The listing builds one solid part. Answer for the finished solid, in the listing's coordinates (mm). A direction names the side the tool comes from. Coordinates: 2 decimals unless noted, no trailing zeros. Write each loop counter-clockwise with the first axis right and the second up, starting at its lowest first coordinate (ties: lowest second). Pieces come first, ordered by that corner, then holes. Notation, with made-up numbers: M 63,82 L 83,82 A31 cw 83,120 Z; hole C 61,-10.5 d10. An arc over 180 degrees is marked long. Answer as CSV lines item,"result". Start each with the question number.
```python
from build123d import *

# Parameters (mm, degrees)
SKETCH1_R           = 9.525
BOSS_EXTRUDE1_DEPTH = 7.62


with BuildPart() as part:
    # Sketch1 → Boss-Extrude1 (new body)
    with BuildSketch(Plane(origin=(0, 0, 0), x_dir=(1, 0, 0), z_dir=(0, 1, 0))):
        with BuildLine():
            Line((-4.826, 49.377023111), (-4.826, 76.047023111))
            ThreePointArc((-4.826, 76.047023111), (-8.902418576, 75.678180102), (-12.953151139, 75.090983983))
            ThreePointArc((-12.953151139, 75.090983983), (-31.496, 54.552672235), (-58.554124155, 48.763249937))
            ThreePointArc((-58.554124155, 48.763249937), (-61.088017192, 45.548810693), (-63.445653896, 42.202950154))
            Line((-63.445653896, 42.202950154), (-40.348756377, 28.867950154))
            ThreePointArc((-40.348756377, 28.867950154), (-38.582317778, 22.275511555), (-45.174756377, 20.509072957))
            Line((-45.174756377, 20.509072957), (-68.271653896, 33.844072957))
            ThreePointArc((-68.271653896, 33.844072957), (-69.990435768, 30.129369409), (-71.507275294, 26.327734046))
            ThreePointArc((-71.507275294, 26.327734046), (-62.992, 0), (-71.507275294, -26.327734046))
            ThreePointArc((-71.507275294, -26.327734046), (-69.990435768, -30.129369409), (-68.271653896, -33.844072957))
            Line((-68.271653896, -33.844072957), (-45.174756377, -20.509072957))
            ThreePointArc((-45.174756377, -20.509072957), (-38.582317778, -22.275511555), (-40.348756377, -28.867950154))
            Line((-40.348756377, -28.867950154), (-63.445653896, -42.202950154))
            ThreePointArc((-63.445653896, -42.202950154), (-61.088017192, -45.548810693), (-58.554124155, -48.763249937))
            ThreePointArc((-58.554124155, -48.763249937), (-31.496, -54.552672235), (-12.953151139, -75.090983983))
            ThreePointArc((-12.953151139, -75.090983983), (-8.902418576, -75.678180102), (-4.826, -76.047023111))
            Line((-4.826, -76.047023111), (-4.826, -49.377023111))
            ThreePointArc((-4.826, -49.377023111), (0, -44.551023111), (4.826, -49.377023111))
            Line((4.826, -49.377023111), (4.826, -76.047023111))
            ThreePointArc((4.826, -76.047023111), (8.902418576, -75.678180102), (12.953151139, -75.090983983))
            ThreePointArc((12.953151139, -75.090983983), (31.496, -54.552672235), (58.554124155, -48.763249937))
            ThreePointArc((58.554124155, -48.763249937), (61.088017192, -45.548810693), (63.445653896, -42.202950154))
            Line((63.445653896, -42.202950154), (40.348756377, -28.867950154))
            ThreePointArc((40.348756377, -28.867950154), (38.582317778, -22.275511555), (45.174756377, -20.509072957))
            Line((45.174756377, -20.509072957), (68.271653896, -33.844072957))
            ThreePointArc((68.271653896, -33.844072957), (69.990435768, -30.129369409), (71.507275294, -26.327734046))
            ThreePointArc((71.507275294, -26.327734046), (62.992, 0), (71.507275294, 26.327734046))
            ThreePointArc((71.507275294, 26.327734046), (69.990435768, 30.129369409), (68.271653896, 33.844072957))
            Line((68.271653896, 33.844072957), (45.174756377, 20.509072957))
            ThreePointArc((45.174756377, 20.509072957), (38.582317778, 22.275511555), (40.348756377, 28.867950154))
            Line((40.348756377, 28.867950154), (63.445653896, 42.202950154))
            ThreePointArc((63.445653896, 42.202950154), (61.088017192, 45.548810693), (58.554124155, 48.763249937))
            ThreePointArc((58.554124155, 48.763249937), (31.496, 54.552672235), (12.953151139, 75.090983983))
            ThreePointArc((12.953151139, 75.090983983), (8.902418576, 75.678180102), (4.826, 76.047023111))
            Line((4.826, 76.047023111), (4.826, 49.377023111))
            ThreePointArc((4.826, 49.377023111), (0, 44.551023111), (-4.826, 49.377023111))
        make_face()
        with Locations(Location((0, 0, 0), (0, 0, 90))):
            Circle(SKETCH1_R, mode=Mode.SUBTRACT)
    extrude(amount=BOSS_EXTRUDE1_DEPTH)


solid = part.part
```
1) Find the intervals of material crossed by line 1 (Z direction, x = -48.5, y = 3); line 2 (Z direction, x = 46.5, y = 4.5); line 3 (X direction, y = 0.75, z = 26), in increasing order. Write a range as from..to.
2) The part is cut by section C-C (z = 23.5). Determine the outline of the cut face in (x, y), then the cut area to 3 significant figures.
3) The part is cut by section D-D (x = -50). Determine the outline of the cut face in (y, z), then the cut area to 3 significant figures.
4) The part is cut by section B-B (z = 0). Determine the outline of the cut face in (x, y) (3 decimals).
5) Which of the six approach directions +Z, -Z, +X, -X, +Y, -Y give full straight-line access (tool end or side, diameter ignored) to faces 5 (the face through (-61.054, 3.757, -45.595)), 6 (the face through (-56.885, 3.757, 27.27)), 7 (the face through (-4.826, 4, -63))?
6) Each of these flat-tipped pins is pushed along its axis until it touches: P1, Ø4, axis at y = 4.5, z = 27, coming from the +X side; P2, Ø4, axis at y = 6, z = 59, coming from the +X side; P3, Ø1, axis at y = 2.5, z = -24.5, coming from the +X side. Where does it stop, or does it pass through?
7) The part is cut by section A-A (x = 0). Determine the outline of the cut face in (y, z) (3 decimals), then the cut area to 3 significant figures.
8) For a pull along X with two mould halves and no side action, classify faces 1 (the face through (-61.122, 3.757, 45.503)), 2 (the face through (38.53, 3.76, 22.37)), 3 (the face through (70.01, 3.76, -30.08)), 4 (the face through (5.796, 3.757, 7.559)) as +X half, -X half, draft (parallel to the pull), parting line (faces both ways), or undercut.
Completed:
1,line 1,"-48.86..-33.57, -22.43..22.43, 33.57..48.86"
1,line 2,"-49.16..-32.42, -21.27..21.27, 32.42..49.16"
1,line 3,"-71.27..-54.69, -38.12..38.12, 54.69..71.27"
2,outline,"M -69.62,0 L -50.36,0 L -50.36,7.62 L -69.62,7.62 Z; M -38.08,0 L 38.08,0 L 38.08,7.62 L -38.08,7.62 Z; M 50.36,0 L 69.62,0 L 69.62,7.62 L 50.36,7.62 Z"
2,area,"874 mm²"
3,outline,"M 0,-48.71 L 7.62,-48.71 L 7.62,-34.44 L 0,-34.44 Z; M 0,-23.29 L 7.62,-23.29 L 7.62,23.29 L 0,23.29 Z; M 0,34.44 L 7.62,34.44 L 7.62,48.71 L 0,48.71 Z"
3,area,"572 mm²"
4,outline,"M -62.992,0 L -9.525,0 L -9.525,7.62 L -62.992,7.62 Z; M 9.525,0 L 62.992,0 L 62.992,7.62 L 9.525,7.62 Z"
5,face 5,"-Z, -X, +Y, -Y"
5,face 6,"+Y, -Y"
5,face 7,"-Z, +Y, -Y"
6,P1,"x = 71.51"
6,P2,"x = 27.71"
6,P3,"x = 70.58"
7,outline,"M 0,-44.551 L 7.62,-44.551 L 7.62,-9.525 L 0,-9.525 Z; M 0,9.525 L 7.62,9.525 L 7.62,44.551 L 0,44.551 Z"
7,area,"534 mm²"
8,face 1,"-X half"
8,face 2,"undercut"
8,face 3,"+X half"
8,face 4,"undercut"
